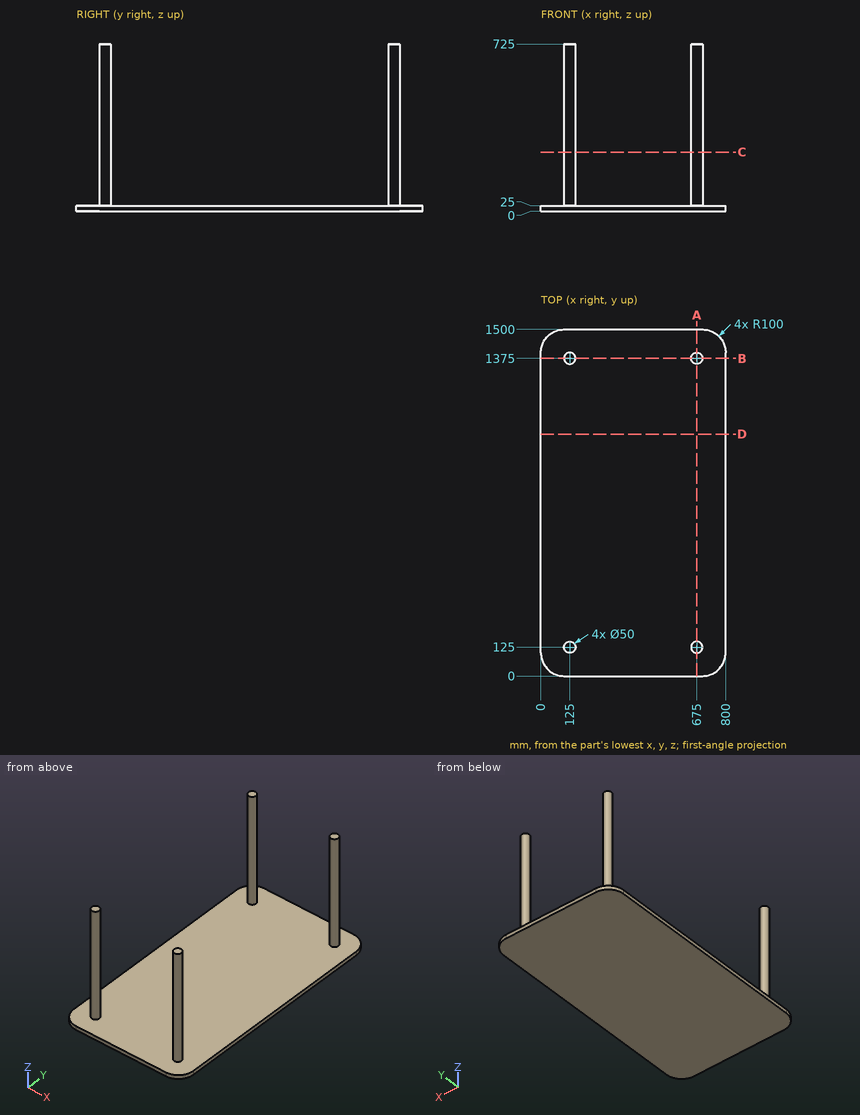
Can you work these out from the drawing? Everything is in mm from the part's minimum corner. Round coordinates to 2 decimals unless told otherwise and drop trailing zeros. Loops run counter-clockwise (first coordinate to the right, second up) from the corner with the lowest first, then second, coordinate; pieces in that order, holes last. Notation, with made-up numbers: (11.25, -36.5) -> (27.25, -36.5) arc R27 cw to (27.25, -5.5) -> close; hole circle Ø7 at (-10, 61). An arc over 180 degrees is marked (long way). Answer in a Markdown table with one row per item.
Item 1: If I drill on probe 1 along Z at (x, y) = (165.5, 1037.5); probe 2 along Y at (x, z) = (120, 231); probe 3 along Y at (x, z) = (688.5, 238), over which ranges is the centre line in solid material (lowest first)?
Answer block:
| item | result |
|---|---|
| probe 1 | 0 to 25 |
| probe 2 | 100.51 to 149.49, 1350.51 to 1399.49 |
| probe 3 | 103.96 to 146.04, 1353.96 to 1396.04 |
Item 2: Suppose I cut it at B-B, the plane y = 1375. List the corners of the cut face in (x, z) for me, plus the area to 3 significant figures.
Answer block:
| item | result |
|---|---|
| outline | (0, 0) -> (800, 0) -> (800, 25) -> (700, 25) -> (700, 725) -> (650, 725) -> (650, 25) -> (150, 25) -> (150, 725) -> (100, 725) -> (100, 25) -> (0, 25) -> close |
| area | 90,000 mm² |
Item 3: Suppose I cut it at A-A, the plane x = 675. List the corners of the cut face in (y, z) for me.
Answer block:
| item | result |
|---|---|
| outline | (0, 0) -> (1500, 0) -> (1500, 25) -> (1400, 25) -> (1400, 725) -> (1350, 725) -> (1350, 25) -> (150, 25) -> (150, 725) -> (100, 725) -> (100, 25) -> (0, 25) -> close |
Item 4: Suppose I cut it at D-D, the plane y = 1047.5. List the corners of the cut face in (x, z) for me, plus the area to 3 significant figures.
Answer block:
| item | result |
|---|---|
| outline | (0, 0) -> (800, 0) -> (800, 25) -> (0, 25) -> close |
| area | 20,000 mm² |
Item 5: Will these pins go through, and if not, where does the flat tip stop? P1, Ø10, axis at x = 684.5, y = 847.5, coming from the -Z side; P2, Ø5, axis at x = 189.5, y = 873.5, coming from the +Z side.
Answer block:
| item | result |
|---|---|
| P1 | z = 0 |
| P2 | z = 25 |
Item 6: Suppose I cut it at C-C, the plane z = 257. List the corners of the cut face in (x, y) for me.
Answer block:
| item | result |
|---|---|
| outline | circle Ø50 at (125, 125); circle Ø50 at (125, 1375); circle Ø50 at (675, 125); circle Ø50 at (675, 1375) |
